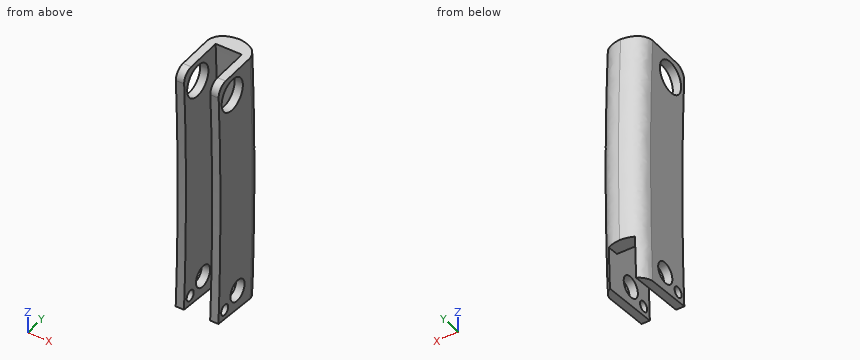
from build123d import *

# Parameters (mm, degrees)
SKETCH4_R          = 1.5
SKETCH4_R_2        = 1
CUT_EXTRUDE1_DEPTH = 23
FILLET1_R          = 1
SKETCH5_R          = 0.5
CUT_EXTRUDE2_DEPTH = 23
SKETCH6_W          = 2.449612404
SKETCH6_H          = 5.085440949
CUT_EXTRUDE3_DEPTH = 4


with BuildPart() as part:
    # Sweep1: sweep along a path in Sketch2
    with BuildLine() as sweep1_path:  # in the path sketch's own coordinates; laid on its plane below (add() does not lay a ready-made edge on the line's plane)
        add(Edge.make_bspline(
            [(0, 0), (12.002417385, 0.593156544), (24, 0)],
            knots=[0, 0, 0, 1, 1, 1], degree=2))
    # Sketch1 → Sweep1 (sweep)
    with BuildSketch(Plane.XY):
        with BuildLine():
            Line((-1.224806202, 0), (1.224806202, 0))
            Line((1.224806202, 0), (1.224806202, -4.5))
            Line((1.224806202, -4.5), (2, -4.5))
            Line((2, -4.5), (2, 0))
            add(Edge.make_bspline(
                [(2, 0), (1.789237919, 1.363268396), (0, 1.5)],
                knots=[0, 0, 0, 1, 1, 1], degree=2))
            add(Edge.make_bspline(
                [(-2, 0), (-1.789237919, 1.363268396), (0, 1.5)],
                knots=[0, 0, 0, 1, 1, 1], degree=2))
            Line((-2, 0), (-2, -4.5))
            Line((-2, -4.5), (-1.224806202, -4.5))
            Line((-1.224806202, -4.5), (-1.224806202, 0))
        make_face()
    sweep(path=Plane(origin=(0, 0, 0), x_dir=(0, 0, -1), z_dir=(1, 0, 0)) * sweep1_path.line)

    # Sketch4 → Cut-Extrude1 (cut)
    with BuildSketch(Plane(origin=(2, 0, 0), x_dir=(0, 0, -1), z_dir=(1, 0, 0))):
        with Locations((2, -2.524194964)):
            Circle(SKETCH4_R)
        with Locations((22, -1.784311687)):
            Circle(SKETCH4_R_2)
    extrude(amount=-CUT_EXTRUDE1_DEPTH, mode=Mode.SUBTRACT)

    # Fillet1
    fillet1_edges = [part.edges().sort_by_distance(p)[0] for p in [
        (-1.612403101, -4.5, 0),
        (1.612403101, -4.5, 0),
    ]]
    fillet(fillet1_edges, radius=FILLET1_R)

    # Sketch5 → Cut-Extrude2 (cut)
    with BuildSketch(Plane(origin=(2, 0, 0), x_dir=(0, 0, -1), z_dir=(1, 0, 0))):
        with Locations((22.73074773, -3.597243091)):
            Circle(SKETCH5_R)
    extrude(amount=-CUT_EXTRUDE2_DEPTH, mode=Mode.SUBTRACT)

    # Sketch6 → Cut-Extrude3 (cut)
    with BuildSketch(Plane(origin=(0, -2.35530576, -23.766585519), x_dir=(-1, 0, 0), z_dir=(0, -0.09861847381015884, -0.9951253170447204))):
        with Locations((0, 3.230896736)):
            Rectangle(SKETCH6_W, SKETCH6_H)
    extrude(amount=-CUT_EXTRUDE3_DEPTH, mode=Mode.SUBTRACT)


solid = part.part
Could you check a few things on this model? Use its own coordinates, in mm. Give positions to 0.01 mm unless a question says otherwise; leave off trailing zeros.
1. Suppose I cut it at A-A (z = -22). Give the number of separate pieces and of enclosed holes in the cut face, plus the area to 3 significant figures.
2. I need wall thicknesses on L1, parallel to X at y = -0.5, z = -18.75; L2, parallel to Z at x = 1.35, y = -2.5; L3, parallel to Y at x = 1.15, z = -12.5. Which ranges of each line are inside material? Lowest first, please.
3. Will this pin go through, and if not, where does the flat tip stop? P1, Ø1.8, axis at y = -1.78, z = -22, coming from the +X side.
Solved:
1. separate pieces: 4
1. enclosed holes: 0
1. area: 5.09 mm2
2. L1: x = -2 to -1.22, 1.22 to 2
2. L2: z = -23.75 to -22.7, -21.3 to -3.5, -0.5 to 0
2. L3: y = 0.3 to 1.5
3. P1: passes through
